For this review, take the finished solid that the model builds, in its own axes (mm). Face numbers are marked on the shaded views. Round coordinates to 2 decimals unless told otherwise and drop trailing zeros. Loops run counter-clockwise (first coordinate to the right, second up) from the corner with the lowest first, then second, coordinate; pieces in that order, holes last.
1. Consider section B-B on z = 3. State the section outline as (x, y) points, then the cut area to 3 significant figures.
2. To check wall thickness, follow line 1 along Y through (x, z) = (-13.5, 17); line 2 along Z through (x, y) = (-38.5, 4.5); line 3 along Y through (x, z) = (-84, 19). State the ranges of each line that lie inside material, in increasing order.
3. Consider section A-A on x = -52. State the section outline as (y, z) points (3 decimals), then the cut area to 3 significant figures.
4. Draft analysis for pull direction Y (two halves, no side actions). For the marked faces 1, 2 and 3, state which applies: released by +Y, released by -Y, zero draft, split by the parting line, or undercut.
5. Consider section C-C on y = 44.5. State the section outline as (x, z) points, then the cut area to 3 significant figures.
6. Clearance check with flat-ended pins moving along their axes: pin 1 Ø1 at (y, z) = (34.5, 15) entering from +X; pin 2 Ø1.9 at (x, y) = (-44.5, 3) entering from -Z; pin 3 Ø6.5 at (x, z) = (-49, 8) entering from +Y. State where each tip first meets the part, or that it passes through.
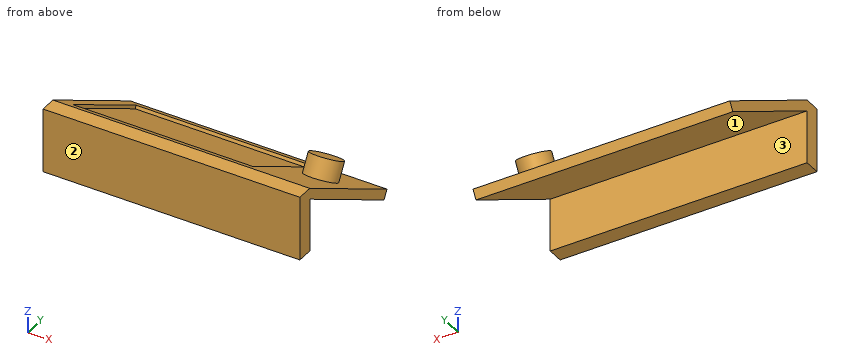
from build123d import *

# Parameters (mm, degrees)
SKETCH1_W           = 101.6
SKETCH1_H           = 6.35
BOSS_EXTRUDE1_DEPTH = 25.4
BOSS_EXTRUDE2_DEPTH = 101.6
SKETCH3_W           = 71.12
SKETCH3_H           = 46.99
CUT_EXTRUDE1_DEPTH  = 1.27
SKETCH4_R           = 6.35
BOSS_EXTRUDE3_DEPTH = 7.62


with BuildPart() as part:
    # Sketch1 → Boss-Extrude1 (new body)
    with BuildSketch(Plane.XY):
        with Locations((-50.8, 3.175)):
            Rectangle(SKETCH1_W, SKETCH1_H)
    extrude(amount=BOSS_EXTRUDE1_DEPTH)

    # Sketch2 → Boss-Extrude2 (add)
    with BuildSketch(Plane(origin=(0, 0, 0), x_dir=(0, 0, -1), z_dir=(1, 0, 0))):
        Polygon((-25.4, 6.35), (3.175, 55.843351826), (6.474556788, 53.938351826), (-21.000590949, 6.35), align=None)
    extrude(amount=-BOSS_EXTRUDE2_DEPTH)

    # Sketch3 → Cut-Extrude1 (cut)
    with BuildSketch(Plane(origin=(0, 12.586022628, 21.799630657), x_dir=(1, 0, 0), z_dir=(0, 0.5, 0.866025404))):
        with Locations((-60.96, 21.374261314)):
            Rectangle(SKETCH3_W, SKETCH3_H)
    extrude(amount=-CUT_EXTRUDE1_DEPTH, mode=Mode.SUBTRACT)

    # Sketch4 → Boss-Extrude3 (add)
    with BuildSketch(Plane(origin=(0, 12.586022628, 21.799630657), x_dir=(1, 0, 0), z_dir=(0, 0.5, 0.866025404))):
        with Locations((-12.7, 24.549261314)):
            Circle(SKETCH4_R)
    extrude(amount=BOSS_EXTRUDE3_DEPTH)


solid = part.part
Resolved:
1. outline: (-101.6, 0) - (0, 0) - (0, 6.35) - (-101.6, 6.35) - close; (-101.6, 37.53) - (0, 37.53) - (0, 45.15) - (-25.4, 45.15) - (-25.4, 42.61) - (-96.52, 42.61) - (-96.52, 45.15) - (-101.6, 45.15) - close
1. area: 1,240 mm2
2. line 1: y = 0 to 6.35, 13.28 to 20.9, 30.89 to 36.14
2. line 2: z = 0 to 25.4
2. line 3: y = 0 to 6.35, 9.82 to 14.9
3. outline: (0, 0) - (6.35, 0) - (6.35, 21.001) - (53.938, -6.475) - (55.843, -3.175) - (51.444, -0.635) - (50.809, -1.735) - (10.114, 21.76) - (10.749, 22.86) - (6.35, 25.4) - (0, 25.4) - close
3. area: 315 mm2
4. face 1: undercut
4. face 2: released by -Y
4. face 3: undercut
5. outline: (-101.6, -1.03) - (0, -1.03) - (0, 3.37) - (-25.4, 3.37) - (-25.4, 1.91) - (-96.52, 1.91) - (-96.52, 3.37) - (-101.6, 3.37) - close
5. area: 343 mm2
6. pin 1: stops at x = -6.57
6. pin 2: stops at z = 0
6. pin 3: stops at y = 39.58
